Can you work these out from the model? Positions are in its coordinate system, mm. Face numbers are marked on the shaded views. Round coordinates to 2 decimals unless told otherwise and drop trailing zeros. Write each loop counter-clockwise with the first axis right and the second up, starting at its lowest first coordinate (ties: lowest second). Pieces come first, ordered by that corner, then holes. Notation, with made-up numbers: (19.5, -20.5) -> (61.5, -20.5) arc R19 cw to (61.5, -8.5) -> close; hole circle Ø3 at (-12.75, 63.25). An arc over 180 degrees is marked (long way). Write item = value, one per line. Start each with the question number.
1) Imagine slicing it at B-B, the plane y = 2.25. Please give me the cut outline in (x, z).
2) If I drill on line 1 (X direction, y = 0.8, z = -6.25); line 2 (X direction, y = 1.7, z = 1.25); line 3 (Z direction, x = 6, y = 0.65), over which ranges is the centre line in solid material (lowest first)?
3) Thinking about a two-plate mould opening in X: for the marked faces 1, 2 and 3, which applies, +X half, -X half, draft (parallel to the pull), parting line (faces both ways), or undercut?
4) Imagine slicing it at A-A, the plane x = -7.5. Please give me the cut outline in (y, z).
5) Imagine slicing it at C-C, the plane x = 12.5. Please give me the cut outline in (y, z), then the cut area to 3 significant figures.
6) I'm going to push flat-ended pins straight in: pin 1 (1 mm diameter, centred on x = 2, y = 2.5, fed in from -Z); pin 2 (2.5 mm diameter, centred on x = 12.5, z = -6.25, fed in from +Y); pin 3 (1.5 mm diameter, centred on x = 12, y = 1.5, fed in from +Z). Where does each tip first touch, or does it pass through?
7) Imagine slicing it at D-D, the plane z = -2. Please give me the cut outline in (x, y), then the cut area to 3 significant figures.
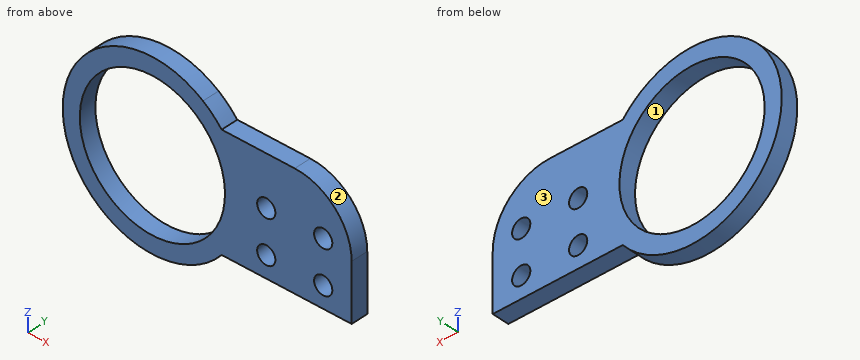
from build123d import *

# Parameters (mm, degrees)
SKETCH_1_W          = 55
SKETCH_1_H          = 20
EXTRUDE_1_DEPTH     = 3
SKETCH_2_R          = 1.6
SKETCH_2_R_2        = 6.75
CUT_EXTRUDE_1_DEPTH = 30.41513216
SKETCH_4_R          = 1.6
CUT_EXTRUDE_2_DEPTH = 30.41513216
EXTRUDE_2_DEPTH     = 3
SKETCH_6_R          = 1.6
CUT_EXTRUDE_3_DEPTH = 31.565503431
SKETCH_7_W          = 8
SKETCH_7_H          = 23
CUT_EXTRUDE_4_DEPTH = 31.565503431
SKETCH_9_R          = 18.063991313
EXTRUDE_4_DEPTH     = 3
SKETCH_10_R         = 12.75
CUT_EXTRUDE_6_DEPTH = 34.038731546
SKETCH_11_OUTSIDE_W = 67.918
SKETCH_11_OUTSIDE_H = 50.982
CUT_EXTRUDE_7_DEPTH = 34.038731546
SKETCH_12_OUTSIDE_W = 64.712
SKETCH_12_OUTSIDE_H = 45.462
CUT_EXTRUDE_8_DEPTH = 32.832569799
FILLET_1_R          = 10


with BuildPart() as part:
    # 草图1 → 凸台-拉伸1 (new body)
    with BuildSketch(Plane(origin=(0, 0, 0), x_dir=(1, 0, 0), z_dir=(0, 1, 0))):
        Rectangle(SKETCH_1_W, SKETCH_1_H)
    extrude(amount=EXTRUDE_1_DEPTH)

    # 草图2 → 切除-拉伸1 (cut, through all)
    with BuildSketch(Plane(origin=(0, 3, 0), x_dir=(1, 0, 0), z_dir=(0, 1, 0))):
        with Locations(Location((-15.727241336, 4.75, 0), (0, 0, 270))):
            Circle(SKETCH_2_R)
        with Locations((-7.5, -9.5)):
            Circle(SKETCH_2_R)
        with Locations(Location((0.727241336, 4.75, 0), (0, 0, 270))):
            Circle(SKETCH_2_R)
        with Locations(Location((-7.5, 0, 0), (0, 0, 270))):
            Circle(SKETCH_2_R_2)
    extrude(amount=-CUT_EXTRUDE_1_DEPTH, mode=Mode.SUBTRACT)

    # 草图4 → 切除-拉伸2 (cut, through all)
    with BuildSketch(Plane(origin=(0, 3, 0), x_dir=(1, 0, 0), z_dir=(0, 1, 0))):
        with Locations(Location((22.5, 6.25, 0), (0, 0, 270))):
            Circle(SKETCH_4_R)
        with Locations(Location((12.5, 6.25, 0), (0, 0, 90))):
            Circle(SKETCH_4_R)
        with Locations(Location((22.5, -1.25, 0), (0, 0, 90))):
            Circle(SKETCH_4_R)
        with Locations(Location((12.5, -1.25, 0), (0, 0, 270))):
            Circle(SKETCH_4_R)
    extrude(amount=-CUT_EXTRUDE_2_DEPTH, mode=Mode.SUBTRACT)

    # 草图5 → 凸台-拉伸2 (add)
    with BuildSketch(Plane(origin=(0, 3, 0), x_dir=(1, 0, 0), z_dir=(0, 1, 0))):
        Polygon((-27.5, -10), (-27.5, -13), (0, -13), (27.5, -13), (27.5, -10), align=None)
    extrude(amount=-EXTRUDE_2_DEPTH)

    # 草图6 → 切除-拉伸3 (cut, through all)
    with BuildSketch(Plane(origin=(0, 3, 0), x_dir=(1, 0, 0), z_dir=(0, 1, 0))):
        with Locations(Location((-7.5, -9.5, 0), (0, 0, 270))):
            Circle(SKETCH_6_R)
    extrude(amount=-CUT_EXTRUDE_3_DEPTH, mode=Mode.SUBTRACT)

    # 草图7 → 切除-拉伸4 (cut, through all)
    with BuildSketch(Plane(origin=(0, 3, 0), x_dir=(1, 0, 0), z_dir=(0, 1, 0))):
        with Locations((-23.5, -1.5)):
            Rectangle(SKETCH_7_W, SKETCH_7_H)
    extrude(amount=-CUT_EXTRUDE_4_DEPTH, mode=Mode.SUBTRACT)

    # 草图9 → 凸台-拉伸4 (add)
    with BuildSketch(Plane(origin=(0, 3, 0), x_dir=(1, 0, 0), z_dir=(0, 1, 0))):
        with Locations((-7.5, 0)):
            Circle(SKETCH_9_R)
    extrude(amount=-EXTRUDE_4_DEPTH)

    # 草图10 → 切除-拉伸6 (cut, through all)
    with BuildSketch(Plane(origin=(0, 3, 0), x_dir=(1, 0, 0), z_dir=(0, 1, 0))):
        with Locations(Location((-7.5, 0, 0), (0, 0, 270))):
            Circle(SKETCH_10_R)
    extrude(amount=-CUT_EXTRUDE_6_DEPTH, mode=Mode.SUBTRACT)

    # 草图11 outside → 切除-拉伸7 (cut, through all)
    with BuildSketch(Plane(origin=(0, 3, 0), x_dir=(1, 0, 0), z_dir=(0, 1, 0))):
        with Locations((0.968, 0)):
            Rectangle(SKETCH_11_OUTSIDE_W, SKETCH_11_OUTSIDE_H)
        with BuildLine():
            Line((27.5, 10), (4.668093524, 10))
            ThreePointArc((4.668093524, 10), (-23.092588853, 2.221187265), (1.391709622, -13))
            Line((1.391709622, -13), (27.5, -13))
            Line((27.5, -13), (27.5, 10))
        make_face(mode=Mode.SUBTRACT)
    extrude(amount=-CUT_EXTRUDE_7_DEPTH, mode=Mode.SUBTRACT)

    # 草图12 outside → 切除-拉伸8 (cut, through all)
    with BuildSketch(Plane(origin=(0, 3, 0), x_dir=(1, 0, 0), z_dir=(0, 1, 0))):
        with Locations((2.125, 0)):
            Rectangle(SKETCH_12_OUTSIDE_W, SKETCH_12_OUTSIDE_H)
        with BuildLine():
            Line((27.5, 10), (27.5, -10))
            Line((27.5, -10), (4.668093524, -10))
            ThreePointArc((4.668093524, -10), (-23.25, 0), (4.668093524, 10))
            Line((4.668093524, 10), (27.5, 10))
        make_face(mode=Mode.SUBTRACT)
    extrude(amount=-CUT_EXTRUDE_8_DEPTH, mode=Mode.SUBTRACT)

    # 圆角1
    fillet_1_edges = [part.edges().sort_by_distance(p)[0] for p in [
        (27.5, 1.5, 10),
    ]]
    fillet(fillet_1_edges, radius=FILLET_1_R)


solid = part.part
Reported:
q1.outline = (4.67, -10) -> (27.5, -10) -> (27.5, 0) arc R10 ccw to (17.5, 10) -> (4.67, 10) arc R15.75 ccw (long way) to start; hole circle Ø25.5 at (-7.5, 0); hole circle Ø3.2 at (12.5, -6.25); hole circle Ø3.2 at (12.5, 1.25); hole circle Ø3.2 at (22.5, -6.25); hole circle Ø3.2 at (22.5, 1.25)
q2.line_1 = -21.96 to -18.61, 3.61 to 10.9, 14.1 to 20.9, 24.1 to 27.5
q2.line_2 = -23.2 to -20.19, 5.19 to 10.9, 14.1 to 20.9, 24.1 to 27.42
q2.line_3 = -10 to 10
q3.face_1 = undercut
q3.face_2 = +X half
q3.face_3 = draft
q4.outline = (0, -15.75) -> (3, -15.75) -> (3, -12.75) -> (0, -12.75) -> close; (0, 12.75) -> (3, 12.75) -> (3, 15.75) -> (0, 15.75) -> close
q5.outline = (0, -10) -> (3, -10) -> (3, -7.85) -> (0, -7.85) -> close; (0, -4.65) -> (3, -4.65) -> (3, -0.35) -> (0, -0.35) -> close; (0, 2.85) -> (3, 2.85) -> (3, 10) -> (0, 10) -> close
q5.area = 40.8 mm²
q6.pin_1 = -12.93
q6.pin_2 = through
q6.pin_3 = 10
q7.outline = (-23.12, 0) -> (-20.09, 0) -> (-20.09, 3) -> (-23.12, 3) -> close; (5.09, 0) -> (27.5, 0) -> (27.5, 3) -> (5.09, 3) -> close
q7.area = 76.3 mm²
